CAD build for the part. Positions are in the model's coordinates, mm. A direction names the side the tool comes from. Round coordinates to 2 decimals unless told otherwise and drop trailing zeros. Order: outer loops, then holes, each group sorted by start corner. A loop starts at its lowest first (then second) coordinate and runs counter-clockwise, first axis right, second up. Notation, with made-up numbers: (50, 30.5) - (90, 30.5) arc R6 ccw to (90, 39.5) - close; hole circle Ø5 at (1.25, 67.5). An arc over 180 degrees is marked (long way). Write item = value, one per line.
Autodesk Inventor part; units mm, degrees
ref_plane "YZ Plane" through (0, 0, 0) normal (1, 0, 0) x (0, 1, 0)
ref_plane "XZ Plane" through (0, 0, 0) normal (0, 1, 0) x (-1, 0, 0)
ref_plane "XY Plane" through (0, 0, 0) normal (0, 0, 1) x (1, 0, 0)
sketch "Эскиз1" plane through (0, 0, 0) normal (0, 1, 0) x (-1, 0, 0)
  line L0 (0, 0) -> (5.5, 0)
  line L1 (5.5, 0) -> (5.5, -35.55)
  line L2 (5.5, -35.55) -> (0, -35.55)
  line L3 (0, -35.55) -> (0, 0)
  line L4 (2.75, 0) -> (2.75, -2.5)
  circle A0 centre (2.75, -2.5) radius 1.85
  dimension "d0" = 5.5
  dimension "d1" = 35.55
  dimension "d4" = 2.5
  dimension "d5" = 3.7
extrude "Выдавливание1" add sketch "Эскиз1" along normal blind 4
fillet "Сопряжение1" radius 2.75 2 edges at (0, 2, 0) (-5.5, 2, 0)
sketch "Эскиз2" plane through (0, 4, 0) normal (0, 1, 0) x (1, 0, 0)
  line L0 (0, 2.75) -> (0, 35.55)
  line L1 (-5.5, 35.55) -> (0, 35.55)
  line L2 (0, 35.55) -> (0, 9.4)
  line L3 (0, 9.4) -> (-5.5, 9.4)
  line L4 (-5.5, 9.4) -> (-5.5, 35.55)
  point P0 (0, 0)
  point P1 (0, 35.55)
  dimension "d7" = 26.15
  dimension "d45" = 32.8
extrude "Выдавливание2" add sketch "Эскиз2" along normal blind 3.7
mirror "Зеркальное отражение3" about plane through (-2.75, 7.7, -22.475) normal (0, 1, 0)
sketch "Эскиз8" plane through (0, 0, -2.75) normal (1, 0, 0) x (0, 0, -1)
  line L0 (0, 0) -> (32.8, 0)
  line L1 (32.8, 0) -> (11.65, 0)
  line L2 (11.65, 0) -> (11.65, 15)
  line L3 (11.65, 15) -> (32.8, 15)
  line L4 (32.8, 15) -> (32.8, 0)
  line L5 (6.65, 4) -> (6.65, 11.4)
  line L6 (11.65, 15) -> (21.65, 15)
  line L7 (21.65, 15) -> (21.65, 11)
  line L8 (21.65, 11) -> (11.65, 11)
  line L9 (11.65, 11) -> (11.65, 15)
  point P0 (-2.75, 0)
  dimension "d35" = 21.15
  dimension "d36" = 15
  dimension "d52" = 26.15
  dimension "d60" = 10
  dimension "d61" = 4
extrude "Выдавливание6" cut sketch "Эскиз8" against normal through all contours L2 L8 L7 L3 L4 L0
sketch "Эскиз13" plane through (-5.5, 15.4, -35.55) normal (0, 1, 0) x (1, 0, 0)
  line L0 (0, 0) -> (0, -11.15)
  line L1 (5.5, 0) -> (0, 0)
  line L2 (5.5, -11.15) -> (5.5, 0)
  line L3 (5.5, -11.15) -> (0, -11.15)
  point P0 (5.5, -35.55)
extrude "Выдавливание11" add sketch "Эскиз13" along normal blind 3
mirror "Зеркальное отражение6" about plane through (0, 0, -35.55) normal (0, 0, -1)
fillet "Сопряжение5" radius 5 12 edges at (-2.75, 0, -14.4) (-2.75, 0, -56.7) (-2.75, 11, -14.4) (-2.75, 11, -24.4) (-2.75, 15, -24.4) (-2.75, 11, -56.7) (-2.75, 11, -46.7) (-2.75, 15, -46.7) (-2.75, 18.4, -24.4) (-2.75, 18.4, -46.7) (-2.75, 15.4, -24.4) (-2.75, 15.4, -46.7)
sketch "Эскиз9" plane through (-2.75, 18.4, 16.75) normal (0, 1, 0) x (1, 0, 0)
  circle A0 centre (0, 52.3) radius 4
  line L0 (-2.75, 58.551) -> (-2.75, 46.049)
  line L1 (-2.75, 52.3) -> (2.75, 52.3)
  line L2 (2.75, 58.551) -> (2.75, 46.049)
  point P0 (2.75, 104.6)
  point P1 (-2.75, 104.6)
  point P2 (60.3162, 64.5588)
  point P3 (0, 52.3)
  dimension "d46" = 8
extrude "Выдавливание7" add sketch "Эскиз9" against normal up to surface (3.4 mm away)
sketch "Эскиз10" plane through (-2.75, 18.4, 16.75) normal (0, 1, 0) x (1, 0, 0)
  arc A0 (-2.75, 55.2047) -> (-2.75, 49.3953) centre (0, 52.3) ccw
  arc A1 (-2.75, 55.2047) -> (-2.75, 49.3953) centre (0, 52.3) ccw
  circle A2 centre (0, 52.3) radius 2.75
  point P0 (2.75, 16.75)
  point P1 (-2.75, 23.7297)
  point P2 (-2.75, 17.9203)
  point P3 (2.75, 17.9203)
  point P4 (2.75, 23.7297)
  dimension "d49" = 5.5
extrude "Выдавливание8" cut sketch "Эскиз10" against normal blind 2.5
properties part number "Балка рулевого управления"
(1) Probe line 1 along X through (y, z) = (17.5, -35.55); line 2 along Z through (x, y) = (-2.75, 1.5); line 3 along Z through (x, y) = (-3, 12.75). List the from-to ranges inside material, lowest first.
Solved:
line_1 = -6.75 to -5.5, 0 to 1.25
line_2 = -71.1 to -70.45, -66.75 to -58.13, -12.97 to -4.35, -0.65 to 0
line_3 = -71.09 to -70.43, -66.77 to -46, -25.1 to -4.33, -0.67 to -0.01
(2) Band-saw the part on C-C on z = -35.55. List the corners of the cut face in (x, y).
Solved:
outline = (-6.75, 15) - (1.25, 15) - (1.25, 18.4) - (0, 18.4) - (0, 15.9) - (-5.5, 15.9) - (-5.5, 18.4) - (-6.75, 18.4) - close
(3) Band-saw the part on A-A on z = -6.5. List the corners of the cut face in (x, y), plus the area to 3 significant figures.
Solved:
outline = (-5.5, 0) - (0, 0) - (0, 4) - (-5.5, 4) - close; (-5.5, 11.4) - (0, 11.4) - (0, 15.4) - (-5.5, 15.4) - close
area = 44.0 mm²
(4) Band-saw the part on D-D on x = -2. Count the separate pieces of the cut face and the enclosed holes in it, plus the area to 3 significant figures.
Solved:
separate_pieces = 5
enclosed_holes = 0
area = 412 mm²
(5) Pull direction Y, two halves, no side cores. Call faces 1 (the flat face through (-3, 11, -20)), 2 (the flat face through (0, 18.4, -34)), 3 (the cylindrical face through (-4.72, 2.03, -0.83)), 4 (the flat face through (-3, 8, -61.7)): released by +Y, released by -Y, zero draft, split by the parting line, or undercut.
Solved:
face_1 = released by -Y
face_2 = released by +Y
face_3 = zero draft
face_4 = undercut
(6) Drop flat-ended pins along their axis: pin 1 (3 mm diameter, centred on y = 7, z = -18, fed in from -X); pin 2 (5 mm diameter, centred on y = 10.5, z = -20, fed in from +X); pin 3 (1.5 mm diameter, centred on x = -6, y = 12.5, fed in from -Z); pin 4 (1.5 mm diameter, centred on x = 0, y = 2.5, fed in from +Z). Give the stop position or say it passes through.
Solved:
pin_1 = through
pin_2 = 0
pin_3 = -69.5
pin_4 = -0.86
(7) Band-saw the part on B-B on y = 8.75. List the corners of the cut face in (x, z).
Solved:
outline = (-5.5, -61.7) - (0, -61.7) - (0, -55.88) - (-5.5, -55.88) - close; (-5.5, -15.22) - (0, -15.22) - (0, -9.4) - (-5.5, -9.4) - close
(8) Tool access for faces 5 (the flat face through (-5.5, 11, -14)), 6 (the flat face through (-3, 15.9, -36)), 7 (the flat face through (-3, 15, -35)), 8 (the flat face through (-3, 8, -9.4)): list every direction of +Z, -Z, +X, -X, +Y, -Y with a clear straight run to the whole face (end or side of a thin tool).
Solved:
face_5 = +Z, -X, +Y, -Y
face_6 = +Y
face_7 = +X, -X, -Y
face_8 = +Z, +X, -X
